from build123d import *

# Parameters (mm, degrees)
SKETCH_1_W               = 60
SKETCH_1_H               = 78
EXTRUDE_1_DEPTH          = 2
SKETCH_2_R               = 2.1
CUT_EXTRUDE_1_DEPTH      = 12
EXTRUDE_2_DEPTH          = 2
SKETCH_4_R               = 1.6
CUT_EXTRUDE_2_DEPTH      = 126
SKETCH_5_R               = 1.946941413
CUT_EXTRUDE_3_DEPTH      = 10
SKETCH_6_R               = 4
SKETCH_6_R_2             = 2.1
EXTRUDE_3_DEPTH          = 5
FILLET_1_R               = 2
SKETCH_8_R               = 2.5
CUT_EXTRUDE_5_DEPTH      = 113
SKETCH_9_R               = 3
CUT_EXTRUDE_6_DEPTH      = 4
SKETCH_11_R              = 2.9
CUT_EXTRUDE_8_DEPTH      = 3.3
MIRROR_3_COPY_1_SKETCH_R = 2.9
MIRROR_3_COPY_1_DEPTH    = 3.3
SKETCH_12_R              = 2.9
CUT_EXTRUDE_9_DEPTH      = 87
SKETCH_13_R              = 2.9
CUT_EXTRUDE_10_DEPTH     = 87


with BuildPart() as part:
    # 草图1 → 凸台-拉伸1 (new body)
    with BuildSketch(Plane(origin=(0, 0, 0), x_dir=(1, 0, 0), z_dir=(0, 1, 0))):
        Rectangle(SKETCH_1_W, SKETCH_1_H)
    extrude(amount=EXTRUDE_1_DEPTH)

    # 草图2 → 切除-拉伸1 (cut)
    with BuildSketch(Plane(origin=(0, 2, 0), x_dir=(1, 0, 0), z_dir=(0, 1, 0))):
        with Locations(Location((-24.5, 17, 0), (0, 0, 270))):
            Circle(SKETCH_2_R)
        with Locations(Location((9.5, 17, 0), (0, 0, 270))):
            Circle(SKETCH_2_R)
        with Locations(Location((9.5, -17, 0), (0, 0, 90))):
            Circle(SKETCH_2_R)
        with Locations(Location((-24.5, -17, 0), (0, 0, 90))):
            Circle(SKETCH_2_R)
    extrude(amount=-CUT_EXTRUDE_1_DEPTH, mode=Mode.SUBTRACT)

    # 草图3 → 凸台-拉伸2 (add)
    with BuildSketch(Plane.XY.offset(39)):
        Polygon((-30, -9), (-30, 11), (30, 11), (30, -9), (30, -19), (-30, -19), align=None)
    extrude_2 = extrude(amount=-EXTRUDE_2_DEPTH)

    # 镜向1: 凸台-拉伸2 across plane
    add(extrude_2.mirror(Plane.XY))

    # 草图4 → 切除-拉伸2 (cut)
    with BuildSketch(Plane.XY.offset(39)):
        with Locations((-25.5, 7)):
            Circle(SKETCH_4_R)
        with Locations((25.5, 7)):
            Circle(SKETCH_4_R)
        with Locations((-25.5, -13)):
            Circle(SKETCH_4_R)
        with Locations((25.5, -14)):
            Circle(SKETCH_4_R)
    extrude(amount=-CUT_EXTRUDE_2_DEPTH, mode=Mode.SUBTRACT)

    # 草图5 → 切除-拉伸3 (cut)
    with BuildSketch(Plane(origin=(0, 2, 0), x_dir=(1, 0, 0), z_dir=(0, 1, 0))):
        with Locations(Location((-22.5, 32, 0), (0, 0, 270))):
            Circle(SKETCH_5_R)
        with Locations(Location((-7.5, 32, 0), (0, 0, 270))):
            Circle(SKETCH_5_R)
        with Locations(Location((7.5, 32, 0), (0, 0, 270))):
            Circle(SKETCH_5_R)
        with Locations(Location((22.5, 32, 0), (0, 0, 270))):
            Circle(SKETCH_5_R)
        with Locations(Location((22.5, -32, 0), (0, 0, 90))):
            Circle(SKETCH_5_R)
        with Locations(Location((7.5, -32, 0), (0, 0, 90))):
            Circle(SKETCH_5_R)
        with Locations(Location((-7.5, -32, 0), (0, 0, 90))):
            Circle(SKETCH_5_R)
        with Locations(Location((-22.5, -32, 0), (0, 0, 90))):
            Circle(SKETCH_5_R)
    extrude(amount=-CUT_EXTRUDE_3_DEPTH, mode=Mode.SUBTRACT)

    # 草图6 → 凸台-拉伸3 (add)
    # profile 1 of 4: a face of its own
    with BuildSketch(Plane(origin=(0, 2, 0), x_dir=(1, 0, 0), z_dir=(0, 1, 0))):
        with Locations(Location((-24.5, 17, 0), (0, 0, 270))):
            Circle(SKETCH_6_R)
        with Locations(Location((-24.5, 17, 0), (0, 0, 270))):
            Circle(SKETCH_6_R_2, mode=Mode.SUBTRACT)
    # profile 2 of 4: a face of its own
    with BuildSketch(Plane(origin=(0, 2, 0), x_dir=(1, 0, 0), z_dir=(0, 1, 0))):
        with Locations(Location((9.5, 17, 0), (0, 0, 270))):
            Circle(SKETCH_6_R)
        with Locations(Location((9.5, 17, 0), (0, 0, 270))):
            Circle(SKETCH_6_R_2, mode=Mode.SUBTRACT)
    # profile 3 of 4: a face of its own
    with BuildSketch(Plane(origin=(0, 2, 0), x_dir=(1, 0, 0), z_dir=(0, 1, 0))):
        with Locations(Location((-24.5, -17, 0), (0, 0, 270))):
            Circle(SKETCH_6_R)
        with Locations(Location((-24.5, -17, 0), (0, 0, 270))):
            Circle(SKETCH_6_R_2, mode=Mode.SUBTRACT)
    # profile 4 of 4: a face of its own
    with BuildSketch(Plane(origin=(0, 2, 0), x_dir=(1, 0, 0), z_dir=(0, 1, 0))):
        with Locations(Location((9.5, -17, 0), (0, 0, 270))):
            Circle(SKETCH_6_R)
        with Locations(Location((9.5, -17, 0), (0, 0, 270))):
            Circle(SKETCH_6_R_2, mode=Mode.SUBTRACT)
    extrude(amount=-EXTRUDE_3_DEPTH)

    # 圆角1
    fillet_1_edges = [part.edges().sort_by_distance(p)[0] for p in [
        (0, 0, 37),
        (0, 0, -37),
    ]]
    fillet(fillet_1_edges, radius=FILLET_1_R)

    # 草图8 → 切除-拉伸5 (cut)
    with BuildSketch(Plane(origin=(0, 0, -39), x_dir=(-1, 0, 0), z_dir=(0, 0, -1))):
        with Locations((0, -9)):
            Circle(SKETCH_8_R)
    extrude(amount=-CUT_EXTRUDE_5_DEPTH, mode=Mode.SUBTRACT)

    # 草图9 → 切除-拉伸6 (cut)
    with BuildSketch(Plane(origin=(0, 2, 0), x_dir=(1, 0, 0), z_dir=(0, 1, 0))):
        with Locations(Location((-24.5, -17, 0), (0, 0, 270))):
            Circle(SKETCH_9_R)
        with Locations(Location((9.5, -17, 0), (0, 0, 270))):
            Circle(SKETCH_9_R)
        with Locations(Location((-24.5, 17, 0), (0, 0, 270))):
            Circle(SKETCH_9_R)
        with Locations(Location((9.5, 17, 0), (0, 0, 270))):
            Circle(SKETCH_9_R)
    extrude(amount=-CUT_EXTRUDE_6_DEPTH, mode=Mode.SUBTRACT)

    # 草图11 → 切除-拉伸8 (cut)
    with BuildSketch(Plane(origin=(0, 0, -39), x_dir=(-1, 0, 0), z_dir=(0, 0, -1))):
        with Locations((-8, -4.5)):
            Circle(SKETCH_11_R)
    cut_extrude_8 = extrude(amount=-CUT_EXTRUDE_8_DEPTH, mode=Mode.SUBTRACT)

    # 镜向2: 切除-拉伸8 across plane
    add(cut_extrude_8.mirror(Plane(origin=(0, 0, 0), x_dir=(0, 0, 1), z_dir=(1, 0, 0))), mode=Mode.SUBTRACT)

    # 镜向3: 切除-拉伸8 across plane
    add(cut_extrude_8.mirror(Plane.XY), mode=Mode.SUBTRACT)

    # 镜向3 copy 1 sketch → 镜向3 copy 1 (cut)
    with BuildSketch(Plane.XY.offset(39)):
        with Locations((-8, -4.5)):
            Circle(MIRROR_3_COPY_1_SKETCH_R)
    extrude(amount=-MIRROR_3_COPY_1_DEPTH, mode=Mode.SUBTRACT)

    # 草图12 → 切除-拉伸9 (cut)
    with BuildSketch(Plane(origin=(0, 0, -39), x_dir=(-1, 0, 0), z_dir=(0, 0, -1))):
        with Locations((-8, 8.5)):
            Circle(SKETCH_12_R)
    extrude(amount=-CUT_EXTRUDE_9_DEPTH, mode=Mode.SUBTRACT)

    # 草图13 → 切除-拉伸10 (cut)
    with BuildSketch(Plane(origin=(0, 0, -39), x_dir=(-1, 0, 0), z_dir=(0, 0, -1))):
        with Locations((8, 8.5)):
            Circle(SKETCH_13_R)
    extrude(amount=-CUT_EXTRUDE_10_DEPTH, mode=Mode.SUBTRACT)


solid = part.part
For this review, take the finished solid that the model builds, in its own axes (mm). A direction names the side the tool comes from. Give positions to 0.01 mm unless a question says otherwise; leave off trailing zeros. Order: outer loops, then holes, each group sorted by start corner. A loop starts at its lowest first (then second) coordinate and runs counter-clockwise, first axis right, second up. Notation, with made-up numbers: M 22,-25 L 81,-25 A16 cw 81,-18 Z; hole C 64,-6 d10. An arc over 180 degrees is marked long. Answer in a Markdown table with one row per item. Add a question column.
(1) Consider section C-C on x = -14.5. State the section outline as (y, z) points.
(2) Mouldability with a two-part tool opening along Z and no side actions: class faces 1 (the face through (0, -4, 39)), 2 (the face through (-26, -3, 19)), 3 (the face through (20, 11, 38)), 4 (the face through (-22.73, -2.49, 18.13)) as +Z half, -Z half, draft (parallel to the pull), parting line (faces both ways), or undercut.
(3) For faces 5 (the face through (8, -3, -15)), 6 (the face through (-21.8, -1.48, -19.95)), 7 (the face through (10.1, -2.5, -38)), 8 (the face through (12, -2, -16)), list the 3-axis set-ups (+Z, -Z, +X, -X, +Y, -Y) from which the entire face can be reached by the end or side of a thin tool; tool diameter is ignored.
(4) Wall thickness on probe 1 along Z at (x, y) = (20, -8); probe 2 along Y at (x, z) = (-18, -19); probe 3 along Y at (x, z) = (-8, 38.45): over which ranges is each line inside the solid? List them lowest first. Write a range as [from, to].
(5) For pin 1 (5 mm diameter, centred on x = -24.5, z = -17, fed in from -Y); pin 2 (4.5 mm diameter, centred on x = -22.5, z = -32, fed in from +Y); pin 3 (1.5 mm diameter, centred on x = 10.5, z = 16, fed in from +Y), all flat-tipped, find the tip position at first contact; note any pin that passes through.
(6) Consider section B-B on y = 1. Give the number of separate pieces and of enclosed holes in the cut face, and give its area (3 significant figures).
(7) Consider section A-A on z = -32. State the section outline as (x, y) points, and give its area (3 significant figures).
(8) Consider section D-D on x = 21.5. State the section outline as (y, z) points.
Evaluation:
| question | item | result |
|---|---|---|
| 1 | outline | M -19,-39 L 11,-39 L 11,-37 L 2,-37 L 2,37 L 11,37 L 11,39 L -19,39 L -19,37 L -2,37 A2 cw 0,35 L 0,-35 A2 cw -2,-37 L -19,-37 Z |
| 2 | face 1 | +Z half |
| 2 | face 2 | undercut |
| 2 | face 3 | draft |
| 2 | face 4 | undercut |
| 3 | face 5 | +X, -X, -Y |
| 3 | face 6 | -Y |
| 3 | face 7 | -Z |
| 3 | face 8 | +Y |
| 4 | probe 1 | z = [-39, -37], [37, 39] |
| 4 | probe 2 | y = [0, 2] |
| 4 | probe 3 | y = [-19, -7.4], [-1.6, 5.6] |
| 5 | pin 1 | stops at y = -3 |
| 5 | pin 2 | stops at y = 2 |
| 5 | pin 3 | stops at y = -2 |
| 6 | separate pieces | 1 |
| 6 | enclosed holes | 12 |
| 6 | area | 4,470 mm^2 |
| 7 | outline | M -30,0 L -24.45,0 L -24.45,2 L -30,2 Z; M -20.55,0 L -9.45,0 L -9.45,2 L -20.55,2 Z; M -5.55,0 L 5.55,0 L 5.55,2 L -5.55,2 Z; M 9.45,0 L 20.55,0 L 20.55,2 L 9.45,2 Z; M 24.45,0 L 30,0 L 30,2 L 24.45,2 Z |
| 7 | area | 88.8 mm^2 |
| 8 | outline | M -19,-39 L 11,-39 L 11,-37 L 2,-37 L 2,-33.67 L 0,-33.67 L 0,-35 A2 cw -2,-37 L -19,-37 Z; M -19,37 L -2,37 A2 cw 0,35 L 0,33.67 L 2,33.67 L 2,37 L 11,37 L 11,39 L -19,39 Z; M 0,-30.33 L 2,-30.33 L 2,30.33 L 0,30.33 Z |
